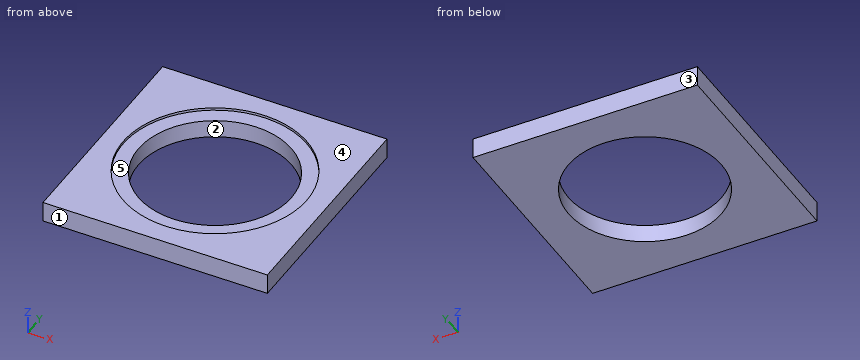
from build123d import *

# Parameters (mm, degrees)
F0_W     = 279.4
F0_H     = 279.4
F1_DEPTH = 25.4
F2_R     = 114.2111
F3_DEPTH = 3.175
F4_R     = 95.1611
F5_DEPTH = 22.225


# Not quite as in the source:
# - a feature of the source that left no trace in its solid (it failed there, or was rolled back) is left out


with BuildPart() as f1:
    # F0 (on Top) → F1 (new body)
    with BuildSketch(Plane.XY):
        Rectangle(F0_W, F0_H)
    extrude(amount=F1_DEPTH)

    # F2 (on face) → F3 (cut)
    with BuildSketch(Plane.XY.offset(25.4)):
        Circle(F2_R)
    extrude(amount=-F3_DEPTH, mode=Mode.SUBTRACT)

    # F4 (on face) → F5 (cut)
    with BuildSketch(Plane.XY.offset(22.225)):
        Circle(F4_R)
    extrude(amount=-F5_DEPTH, mode=Mode.SUBTRACT)


solid = f1.part
Part model, mm, in its own coordinate system. Face numbers are marked on the shaded views. A direction names the side the tool comes from. Give positions to 0.01 mm unless a question says otherwise; leave off trailing zeros. Write each loop counter-clockwise with the first axis right and the second up, starting at its lowest first coordinate (ties: lowest second). Pieces come first, ordered by that corner, then holes.
1) Cut at C-C on z = 15. Write the cut outline in (x, y).
Resolved:
outline: (-139.7, -139.7) - (139.7, -139.7) - (139.7, 139.7) - (-139.7, 139.7) - close; hole circle Ø190.32 at (0, 0)
2) Which spindle directions (+Z, -Z, +X, -X, +Y, -Y) get a long thin tool onto all of the face, cutting with end or side? Do the marked faces 4 and 5. Say none if no direction does.
Resolved:
face 4: +Z, +X, -X, +Y, -Y
face 5: +Z
3) Probe L1, parallel to Y at x = 0, z = 24.6; L2, parallel to Y at x = 3.5, z = 13.5; L3, parallel to X at y = -1, z = 11.5. List the from-to ranges inside material, lowest first.
Resolved:
L1: y = -139.7 to -114.21, 114.21 to 139.7
L2: y = -139.7 to -95.1, 95.1 to 139.7
L3: x = -139.7 to -95.16, 95.16 to 139.7
4) Two-plate mould, pull along Y, no slides. Class the marked faces 1, 2 and 3: released by +Y, released by -Y, zero draft, split by the parting line, or undercut.
Resolved:
face 1: released by -Y
face 2: undercut
face 3: released by +Y
5) Pin check, flat tip, straight feed: pin 1 (12 mm diameter, centred on x = 84.5, y = -11.5, fed in from -Z). Stop position of the tip, or through.
Resolved:
pin 1: passes through
6) Cut at D-D on y = -105.5. Write the cut outline in (x, z) (3 decimals).
Resolved:
outline: (-139.7, 0) - (139.7, 0) - (139.7, 25.4) - (43.748, 25.4) - (43.748, 22.225) - (-43.748, 22.225) - (-43.748, 25.4) - (-139.7, 25.4) - close
7) Cut at A-A on y = 0. Write the cut outline in (x, z) (3 decimals).
Resolved:
outline: (-139.7, 0) - (-95.161, 0) - (-95.161, 22.225) - (-114.211, 22.225) - (-114.211, 25.4) - (-139.7, 25.4) - close; (95.161, 0) - (139.7, 0) - (139.7, 25.4) - (114.211, 25.4) - (114.211, 22.225) - (95.161, 22.225) - close
